from build123d import *

# Parameters (mm, degrees)
BACK_COVER_DEPTH     = 9
COVER_POCKET_DEPTH   = 7
SK_POSTS_R           = 3
SK_POSTS_R_2         = 2.2
IR_BOARD_POSTS_DEPTH = 5
SK_CAP_W             = 26.45
SK_CAP_H             = 2
CABLE_CAP_DEPTH      = 4
SK_CAPSLOT_W         = 23.64
SK_CAPSLOT_H         = 0.59
RIBBON_SLOT_DEPTH    = 4
SK_FINGER1_R         = 1.6
HINGE_FINGER_1_DEPTH = 1.5
SK_FINGER2_R         = 1.6
HINGE_FINGER_2_DEPTH = 1.5
SK_FINGER3_R         = 1.6
HINGE_FINGER_3_DEPTH = 1.5


with BuildPart() as part:
    # Sk_SkirtOuter → Back Cover (new body)
    with BuildSketch(Plane.XY.offset(-4)):
        with BuildLine():
            Line((29.79, 20), (18.34, 20))
            Line((18.34, 20), (18.34, 28))
            Line((18.34, 28), (-20.66, 28))
            Line((-20.66, 28), (-20.66, 20))
            Line((-20.66, 20), (-32.11, 20))
            ThreePointArc((-32.11, 20), (-46.61, 5.5), (-32.11, -9))
            Line((-32.11, -9), (-19.66, -9))
            Line((-19.66, -9), (-19.66, -14))
            Line((-19.66, -14), (17.34, -14))
            Line((17.34, -14), (17.34, -9))
            Line((17.34, -9), (29.79, -9))
            ThreePointArc((29.79, -9), (44.29, 5.5), (29.79, 20))
        make_face()
    extrude(amount=-BACK_COVER_DEPTH)

    # Sk_SkirtInner → Cover Pocket (cut)
    with BuildSketch(Plane.XY.offset(-4)):
        with BuildLine():
            Line((29.79, 18), (16.34, 18))
            Line((16.34, 18), (16.34, 26))
            Line((16.34, 26), (-18.66, 26))
            Line((-18.66, 26), (-18.66, 18))
            Line((-18.66, 18), (-32.11, 18))
            ThreePointArc((-32.11, 18), (-44.61, 5.5), (-32.11, -7))
            Line((-32.11, -7), (-17.66, -7))
            Line((-17.66, -7), (-17.66, -12))
            Line((-17.66, -12), (15.34, -12))
            Line((15.34, -12), (15.34, -7))
            Line((15.34, -7), (29.79, -7))
            ThreePointArc((29.79, -7), (42.29, 5.5), (29.79, 18))
        make_face()
    extrude(amount=-COVER_POCKET_DEPTH, mode=Mode.SUBTRACT)

    # Sk_Posts → IR Board Posts (add)
    # profile 1 of 2: a face of its own
    with BuildSketch(Plane.XY.offset(-6)):
        with Locations((-32.11, 5.5)):
            Circle(SK_POSTS_R)
        with Locations((-32.11, 5.5)):
            Circle(SK_POSTS_R_2, mode=Mode.SUBTRACT)
    # profile 2 of 2: a face of its own
    with BuildSketch(Plane.XY.offset(-6)):
        with Locations((29.79, 5.5)):
            Circle(SK_POSTS_R)
        with Locations((29.79, 5.5)):
            Circle(SK_POSTS_R_2, mode=Mode.SUBTRACT)
    extrude(amount=-IR_BOARD_POSTS_DEPTH)

    # Sk_Cap → Cable Cap (add)
    with BuildSketch(Plane.XY.offset(-7)):
        with Locations((-1.175, 29)):
            Rectangle(SK_CAP_W, SK_CAP_H)
    extrude(amount=-CABLE_CAP_DEPTH)

    # Sk_CapSlot → Ribbon Slot (cut)
    with BuildSketch(Plane.XY.offset(-7)):
        with Locations((-1.18, 28.195)):
            Rectangle(SK_CAPSLOT_W, SK_CAPSLOT_H)
    extrude(amount=-RIBBON_SLOT_DEPTH, mode=Mode.SUBTRACT)

    # Sk_Finger1 → Hinge Finger 1 (add, symmetric)
    with BuildSketch(Plane(origin=(-7.16, 0, 0), x_dir=(0, 0, -1), z_dir=(1, 0, 0))):
        with BuildLine():
            Line((13, -0.88), (20, -0.88))
            ThreePointArc((20, -0.88), (26, 5.12), (20, 11.12))
            Line((20, 11.12), (13, 11.12))
            Line((13, 11.12), (13, -0.88))
        make_face()
        with Locations((20, 5.12)):
            Circle(SK_FINGER1_R, mode=Mode.SUBTRACT)
    extrude(amount=HINGE_FINGER_1_DEPTH, both=True)

    # Sk_Finger2 → Hinge Finger 2 (add, symmetric)
    with BuildSketch(Plane(origin=(-1.16, 0, 0), x_dir=(0, 0, -1), z_dir=(1, 0, 0))):
        with BuildLine():
            Line((13, -0.88), (20, -0.88))
            ThreePointArc((20, -0.88), (26, 5.12), (20, 11.12))
            Line((20, 11.12), (13, 11.12))
            Line((13, 11.12), (13, -0.88))
        make_face()
        with Locations((20, 5.12)):
            Circle(SK_FINGER2_R, mode=Mode.SUBTRACT)
    extrude(amount=HINGE_FINGER_2_DEPTH, both=True)

    # Sk_Finger3 → Hinge Finger 3 (add, symmetric)
    with BuildSketch(Plane(origin=(4.84, 0, 0), x_dir=(0, 0, -1), z_dir=(1, 0, 0))):
        with BuildLine():
            Line((13, -0.88), (20, -0.88))
            ThreePointArc((20, -0.88), (26, 5.12), (20, 11.12))
            Line((20, 11.12), (13, 11.12))
            Line((13, 11.12), (13, -0.88))
        make_face()
        with Locations((20, 5.12)):
            Circle(SK_FINGER3_R, mode=Mode.SUBTRACT)
    extrude(amount=HINGE_FINGER_3_DEPTH, both=True)


solid = part.part
Part model, mm, in its own coordinate system. A direction names the side the tool comes from. Coordinates: 2 decimals unless noted, no trailing zeros. Write each loop counter-clockwise with the first axis right and the second up, starting at its lowest first coordinate (ties: lowest second). Pieces come first, ordered by that corner, then holes. Notation, with made-up numbers: (56.25, 86.5) - (63.25, 86.5) arc R11 cw to (63.25, 101.5) - close; hole circle Ø4 at (28, 1). An arc over 180 degrees is marked (long way). Put each result on its own line as item: value.
1. Band-saw the part on D-D (z = -12). Write the cut outline in (x, y).
Final values:
outline: (-32.11, -9) - (-19.66, -9) - (-19.66, -14) - (17.34, -14) - (17.34, -9) - (29.79, -9) arc R14.5 ccw to (29.79, 20) - (18.34, 20) - (18.34, 28) - (-20.66, 28) - (-20.66, 20) - (-32.11, 20) arc R14.5 ccw to start
2. Flat gauge pins, fed straight in: pin 1 Ø5 at (y, z) = (-1, -16.5) entering from -X; pin 2 Ø1.5 at (x, z) = (6, -20) entering from +Y; pin 3 Ø7 at (x, y) = (29.79, 5.5) entering from +Z; pin 4 Ø1.9 at (y, z) = (5.12, -20) entering from -X. Where does each tip first touch, or does it go through?
Final values:
pin 1: stops at x = -8.66
pin 2: stops at y = 11.12
pin 3: stops at z = -6
pin 4: passes through
3. 3-axis set-ups, long thin cutter, end or side, ignore diameter. For faces 1 (the flat face through (-33, 8, -6)), 2 (the flat face through (17.34, -12, -8)), 3 (the flat face through (-7, -0.88, -16)), 4 (the flat face through (5, 11.12, -17)): which of +Z, -Z, +X, -X, +Y, -Y reach the whole face in a straight line?
Final values:
face 1: +Z
face 2: +Z, -Z, +X, -Y
face 3: -Z, +X, -X, -Y
face 4: -Z, +X, -X, +Y
4. Band-saw the part on A-A (z = -17.5). Write the cut outline in (x, y).
Final values:
outline: (-8.66, -0.88) - (-5.66, -0.88) - (-5.66, 11.12) - (-8.66, 11.12) - close; (-2.66, -0.88) - (0.34, -0.88) - (0.34, 11.12) - (-2.66, 11.12) - close; (3.34, -0.88) - (6.34, -0.88) - (6.34, 11.12) - (3.34, 11.12) - close
5. Probe line 1 along X through (y, z) = (6, -16.75); line 2 along Y through (x, z) = (29.79, -7.4); line 3 along Z through (x, y) = (4, 5). List the from-to ranges inside material, lowest first. Write a range as [from, to].
Final values:
line 1: x = [-8.66, -5.66], [-2.66, 0.34], [3.34, 6.34]
line 2: y = [-9, -7], [2.5, 3.3], [7.7, 8.5], [18, 20]
line 3: z = [-26, -21.6], [-18.4, -11]
6. Two-plate mould, pull along X, no slides. Class faces 5 (the flat face through (-20.66, 24, -8)), 6 (the cylindrical face through (27.592, 5.597, -8.465)), 7 (the cylindrical face through (4.82, 3.56, -19.65)): +X half, -X half, draft (parallel to the pull), parting line (faces both ways), or undercut.
Final values:
face 5: -X half
face 6: undercut
face 7: draft
7. Band-saw the part on C-C (x = -36). Write the cut outline in (y, z), then the cut area to 3 significant figures.
Final values:
outline: (-8.47, -13) - (19.47, -13) - (19.47, -4) - (17.38, -4) - (17.38, -11) - (-6.38, -11) - (-6.38, -4) - (-8.47, -4) - close
area: 85.1 mm²
8. Band-saw the part on B-B (y = -10). Write the cut outline in (x, z).
Final values:
outline: (-19.66, -13) - (17.34, -13) - (17.34, -4) - (15.34, -4) - (15.34, -11) - (-17.66, -11) - (-17.66, -4) - (-19.66, -4) - close
